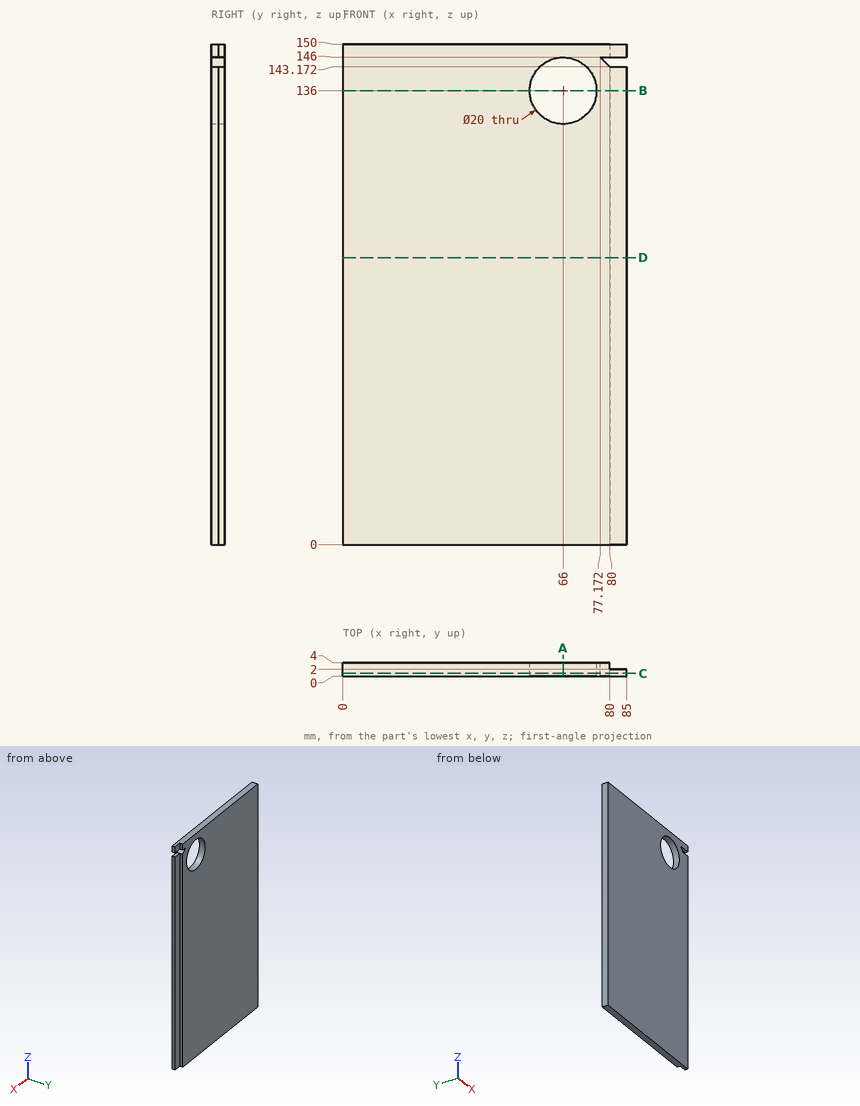
Can you work these out from the drawing? Everything is in mm from the part's minimum corner. Give positions to 0.01 mm unless a question says otherwise; leave off trailing zeros. Order: outer loops, then holes, each group sorted by start corner. A loop starts at its lowest first (then second) coordinate and runs counter-clockwise, first axis right, second up. Notation, with made-up numbers: (43.5, 64) -> (50.5, 64) arc R7 cw to (50.5, 73) -> close; hole circle Ø6 at (75, 82.25). An arc over 180 degrees is marked (long way). Return JSON: item names as keys, results as strings.
1. Imagine slicing it at A-A on x = 66. List the corners of the cut face in (y, z) for me.
Answer list:
{"outline": "(0, 0) -> (4, 0) -> (4, 126) -> (0, 126) -> close; (0, 146) -> (4, 146) -> (4, 150) -> (0, 150) -> close"}
2. Imagine slicing it at D-D on z = 86. List the corners of the cut face in (x, y) for me, then the cut area to 3 significant figures.
Answer list:
{"outline": "(0, 0) -> (85, 0) -> (85, 2) -> (80, 2) -> (80, 4) -> (0, 4) -> close", "area": "330 mm2"}
3. I need wall thicknesses on line 1 (Z direction, x = 66, y = 2.35); line 2 (Z direction, x = 67, y = 3.35); line 3 (X direction, y = 2.7, z = 98). Which ranges of each line are inside material? Lowest first, please. Write a range as from..to.
Answer list:
{"line 1": "z = 0..126, 146..150", "line 2": "z = 0..126.05, 145.95..150", "line 3": "x = 0..80"}
4. Imagine slicing it at B-B on z = 136. List the corners of the cut face in (x, y) for me, then the cut area to 3 significant figures.
Answer list:
{"outline": "(0, 0) -> (56, 0) -> (56, 4) -> (0, 4) -> close; (76, 0) -> (85, 0) -> (85, 2) -> (80, 2) -> (80, 4) -> (76, 4) -> close", "area": "250 mm2"}
5. Imagine slicing it at C-C on y = 0.75. List the corners of the cut face in (x, z) for me.
Answer list:
{"outline": "(0, 0) -> (85, 0) -> (85, 143.17) -> (80, 143.17) -> (77.17, 146) -> (85, 146) -> (85, 150) -> (0, 150) -> close; hole circle Ø20 at (66, 136)"}
6. For pin 1 Ø1.5 at (x, z) = (82, 59) entering from +Y; pin 2 Ø0.6 at (y, z) = (3.5, 148.5) entering from +X, each with a flat end and sliding along its axis, tell me the tip position at first contact or that it passes through.
Answer list:
{"pin 1": "stops at y = 2", "pin 2": "stops at x = 80"}
